Read the model definition and answer for the solid it produces. Units are mm, in the model's axes. A direction names the side the tool comes from. Coordinates: 2 decimals unless noted, no trailing zeros. Loops run counter-clockwise (first coordinate to the right, second up) from the corner with the lowest first, then second, coordinate; pieces in that order, holes last. Notation, with made-up numbers: (-18.75, 67.5) - (19.25, 67.5) arc R30 cw to (19.25, 99.5) - close; hole circle Ø9 at (66.5, 25.5). An arc over 180 degrees is marked (long way). One line per item, written item: value. Start each with the question number.
from build123d import *

# Parameters (mm, degrees)
SKETCH1_W           = 35
SKETCH1_H           = 13
BOSS_EXTRUDE1_DEPTH = 13.5
BOSS_EXTRUDE2_DEPTH = 1.5
BOSS_EXTRUDE3_DEPTH = 1.5
SKETCH4_R           = 1.5
CUT_EXTRUDE1_DEPTH  = 1.5
SKETCH5_W           = 35
SKETCH5_H           = 2.3
CUT_EXTRUDE2_DEPTH  = 6.6
SKETCH6_W           = 10
SKETCH6_H           = 6.2
BOSS_EXTRUDE4_DEPTH = 6.2
SKETCH6_2_W         = 10
SKETCH6_2_H         = 6.2
BOSS_EXTRUDE5_DEPTH = 2.3


with BuildPart() as part:
    # Sketch1 → Boss-Extrude1 (new body)
    with BuildSketch(Plane(origin=(0, 0, 0), x_dir=(1, 0, 0), z_dir=(0, 1, 0))):
        Rectangle(SKETCH1_W, SKETCH1_H)
    extrude(amount=BOSS_EXTRUDE1_DEPTH)

    # Sketch2 → Boss-Extrude2 (add)
    with BuildSketch(Plane.XZ):
        with BuildLine():
            Line((17.5, 3.75), (17.5, -3.75))
            Line((17.5, -3.75), (21.95, -3.75))
            ThreePointArc((21.95, -3.75), (25.7, 0), (21.95, 3.75))
            Line((21.95, 3.75), (17.5, 3.75))
        make_face()
    extrude(amount=-BOSS_EXTRUDE2_DEPTH)

    # Sketch3 → Boss-Extrude3 (add)
    with BuildSketch(Plane.XZ):
        with BuildLine():
            Line((-17.5, 3.75), (-17.5, -3.75))
            Line((-17.5, -3.75), (-21.95, -3.75))
            ThreePointArc((-21.95, -3.75), (-25.7, 0), (-21.95, 3.75))
            Line((-21.95, 3.75), (-17.5, 3.75))
        make_face()
    extrude(amount=-BOSS_EXTRUDE3_DEPTH)

    # Sketch4 → Cut-Extrude1 (cut)
    with BuildSketch(Plane(origin=(0, 1.5, 0), x_dir=(1, 0, 0), z_dir=(0, 1, 0))):
        with Locations(Location((21.95, 0, 0), (0, 0, 270))):
            Circle(SKETCH4_R)
    cut_extrude1 = extrude(amount=-CUT_EXTRUDE1_DEPTH, mode=Mode.SUBTRACT)

    # Mirror1: Cut-Extrude1 across plane
    add(cut_extrude1.mirror(Plane(origin=(0, 0, 0), x_dir=(0, 0, 1), z_dir=(1, 0, 0))), mode=Mode.SUBTRACT)

    # Sketch5 → Cut-Extrude2 (cut)
    with BuildSketch(Plane(origin=(0, 13.5, 0), x_dir=(1, 0, 0), z_dir=(0, 1, 0))):
        with Locations((0, 5.35)):
            Rectangle(SKETCH5_W, SKETCH5_H)
        with Locations((0, -5.35)):
            Rectangle(SKETCH5_W, SKETCH5_H)
    extrude(amount=-CUT_EXTRUDE2_DEPTH, mode=Mode.SUBTRACT)

    # Sketch6 → Boss-Extrude4 (add)
    with BuildSketch(Plane(origin=(0, 0, -6.5), x_dir=(-1, 0, 0), z_dir=(0, 0, -1))):
        with Locations((0, 8)):
            Rectangle(SKETCH6_W, SKETCH6_H)
    extrude(amount=BOSS_EXTRUDE4_DEPTH)

    # Sketch6<2> → Boss-Extrude5 (add)
    with BuildSketch(Plane(origin=(0, 0, -6.5), x_dir=(-1, 0, 0), z_dir=(0, 0, -1))):
        with Locations((0, 8)):
            Rectangle(SKETCH6_2_W, SKETCH6_2_H)
    extrude(amount=-BOSS_EXTRUDE5_DEPTH)


solid = part.part
1) Section C-C, the plane x = 8 is taken. Determine the outline of the cut face in (y, z).
2) For faces 1 (the flat face through (0, 6.9, 5)), 2 (the flat face through (-20, 1.5, 0)), 3 (the flat face through (-20, 1, -3.75)), determine the directions among +Z, -Z, +X, -X, +Y, -Y from which every point of the face is accessible in a straight line to the end or side of a thin tool.
3) Flat-ended cylindrical pins translate along their axes: P1, Ø1.2, axis at x = -20, y = 0.5, coming from the +Z side; P2, Ø2, axis at y = 5.5, z = -3, coming from the -X side; P3, Ø1.9, axis at x = 0, z = -10, coming from the -Y side. Find the tip coordinate at first contact, or state that the pin passes through.
4) Section D-D, the plane z = -8 is taken. Determine the outline of the cut face in (x, y), and give its area (3 significant figures).
5) Section A-A, the plane z = 0 is taken. Determine the outline of the cut face in (x, y), and give its area (3 significant figures).
6) Section B-B, the plane y = 8.5 is taken. Determine the outline of the cut face in (x, z).
7) Determine the mould class of faces 4 (the cylindrical face through (23.437, 0.76, -0.195)), 5 (the cylindrical face through (-25.7, 0.7, -0.1)), 6 (the flat face through (20, 1.5, 0)) for opening direction X: released by +X, released by -X, zero draft, split by the parting line, or undercut.
8) Straight lines are drawn through the part: L1, parallel to X at y = 0.9, z = 0; L2, parallel to Z at x = -21.95, y = 0.9; L3, parallel to X at y = 8, z = -7.5. For each, find the intervals that lie inside material, in ascending order.
Answer below:
1. outline: (0, -6.5) - (6.9, -6.5) - (6.9, -4.2) - (13.5, -4.2) - (13.5, 4.2) - (6.9, 4.2) - (6.9, 6.5) - (0, 6.5) - close
2. face 1: +Z, +X, -X, +Y
2. face 2: +Z, -Z, -X, +Y
2. face 3: -Z, -X, +Y, -Y
3. P1: z = 3.75
3. P2: x = -17.5
3. P3: y = 4.9
4. outline: (-5, 4.9) - (5, 4.9) - (5, 11.1) - (-5, 11.1) - close
4. area: 62.0 mm2
5. outline: (-25.7, 0) - (-23.45, 0) - (-23.45, 1.5) - (-25.7, 1.5) - close; (-20.45, 0) - (20.45, 0) - (20.45, 1.5) - (17.5, 1.5) - (17.5, 13.5) - (-17.5, 13.5) - (-17.5, 1.5) - (-20.45, 1.5) - close; (23.45, 0) - (25.7, 0) - (25.7, 1.5) - (23.45, 1.5) - close
5. area: 488 mm2
6. outline: (-17.5, -4.2) - (-5, -4.2) - (-5, -12.7) - (5, -12.7) - (5, -4.2) - (17.5, -4.2) - (17.5, 4.2) - (-17.5, 4.2) - close
7. face 4: undercut
7. face 5: released by -X
7. face 6: zero draft
8. L1: -25.7 to -23.45, -20.45 to 20.45, 23.45 to 25.7
8. L2: -3.75 to -1.5, 1.5 to 3.75
8. L3: -5 to 5
